Verification items for the finished model (mm, model axes). Face numbers are marked on the shaded views. A direction names the side the tool comes from. Give positions to 0.01 mm unless a question says otherwise; leave off trailing zeros. Order: outer loops, then holes, each group sorted by start corner. A loop starts at its lowest first (then second) coordinate and runs counter-clockwise, first axis right, second up. Notation, with made-up numbers: (-25, 24.5) - (24, 24.5) arc R13 ccw to (24, 39.5) - close; hole circle Ø5 at (73.5, -28). An arc over 180 degrees is marked (long way). Answer as a JSON object with one key per item and string values. Group by question number.
(1) Section check A-A (y = 3.5). Record the boundary of the cut face in (x, z), then the cut area to 3 significant figures.
(2) Mould release check, pull along Y, two halves, no side actions. Record for the marked faces 4, 5, 6 and 7: +Y half, -Y half, draft (parallel to the pull), parting line (faces both ways), or undercut.
(3) Depth check by flat-ended pin: pin 1 Ø12 at (y, z) = (18, -13.5) entering from +X; pin 2 Ø1.5 at (x, y) = (5, -15) entering from +Z; pin 3 Ø0.9 at (y, z) = (13, -18) entering from -X; pin 4 Ø3.5 at (x, y) = (-17.5, 13.5) entering from -Z. Enter the tip coordinate at first touch or a pass-through.
(4) Thickness scan on line 1 (X direction, y = -29, z = -12); line 2 (Z direction, x = 15, y = -28); line 3 (X direction, y = -29, z = -14). Record the ranges inside material, lowest first.
(5) Section check B-B (y = -48). Record the boundary of the cut face in (x, z), then the cut area to 3 significant figures.
(6) Access from +Z, -Z, +X, -X, +Y, -Y to the whole of each face (thin tool, end or side, straight path). Record for the marked faces 1, 2 and 3.
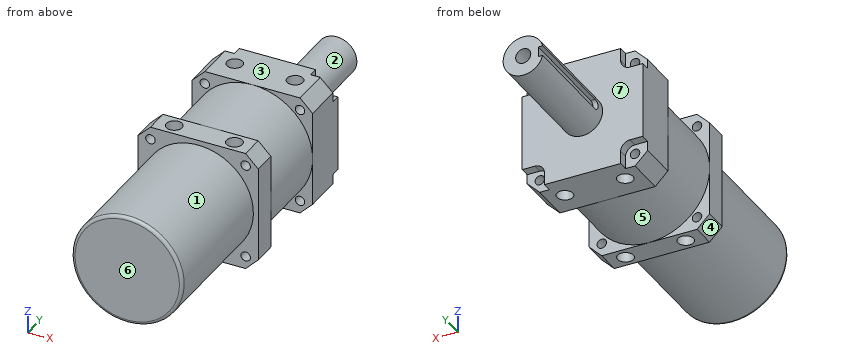
```python
from build123d import *

# Parameters (mm, degrees)
SALIENTE_EXTRUIR1_DEPTH = 15.24
CROQUIS2_R              = 6.35
SALIENTE_EXTRUIR2_DEPTH = 36
CORTAR_EXTRUIR1_DEPTH   = 1.585
CROQUIS4_R              = 1.5
CORTAR_EXTRUIR2_DEPTH   = 58.890781738
CROQUIS5_R              = 19.05
SALIENTE_EXTRUIR3_DEPTH = 25.4
SALIENTE_EXTRUIR4_START = 7.62
CROQUIS6_R              = 1.5
SALIENTE_EXTRUIR4_DEPTH = 7.62
CORTAR_EXTRUIR3_DEPTH   = 3
REDONDEO1_R             = 3
CROQUIS8_R              = 17.5
SALIENTE_EXTRUIR5_DEPTH = 43
REDONDEO2_R             = 1
CROQUIS9_R              = 2.5
CORTAR_EXTRUIR4_DEPTH   = 10
CORTAR_EXTRUIR5_START   = 28.1
CROQUIS9_2_R            = 2.5
CORTAR_EXTRUIR5_DEPTH   = 10
CROQUIS10_R             = 2.3840625
CORTAR_EXTRUIR6_DEPTH   = 15


with BuildPart() as part:
    # Croquis1 → Saliente-Extruir1 (new body)
    with BuildSketch(Plane(origin=(0, 0, 0), x_dir=(1, 0, 0), z_dir=(0, 1, 0))):
        Polygon((-15.05, 19.05), (-19.05, 15.05), (-19.05, -15.05), (-15.05, -19.05), (15.05, -19.05), (19.05, -15.05), (19.05, 15.05), (15.05, 19.05), align=None)
    extrude(amount=SALIENTE_EXTRUIR1_DEPTH)

    # Croquis2 → Saliente-Extruir2 (add)
    with BuildSketch(Plane(origin=(0, 15.24, 0), x_dir=(1, 0, 0), z_dir=(0, 1, 0))):
        with Locations(Location((0, 0, 0), (0, 0, 270))):
            Circle(CROQUIS2_R)
    extrude(amount=SALIENTE_EXTRUIR2_DEPTH)

    # Croquis3 → Cortar-Extruir1 (cut)
    with BuildSketch(Plane.ZY.offset(6.35)):
        with BuildLine():
            Line((-1.5875, 51.24), (-1.5875, 19.49))
            ThreePointArc((-1.5875, 19.49), (-0.0025, 17.905), (1.5825, 19.49))
            Line((1.5825, 19.49), (1.5825, 51.24))
            Line((1.5825, 51.24), (-1.5875, 51.24))
        make_face()
    extrude(amount=-CORTAR_EXTRUIR1_DEPTH, mode=Mode.SUBTRACT)

    # Croquis4 → Cortar-Extruir2 (cut, through all)
    with BuildSketch(Plane.XZ):
        with Locations(Location((-15.05, -15.05, 0), (0, 0, 270))):
            Circle(CROQUIS4_R)
        with Locations(Location((-15.05, 15.05, 0), (0, 0, 270))):
            Circle(CROQUIS4_R)
        with Locations(Location((15.05, 15.05, 0), (0, 0, 270))):
            Circle(CROQUIS4_R)
        with Locations(Location((15.05, -15.05, 0), (0, 0, 270))):
            Circle(CROQUIS4_R)
    extrude(amount=-CORTAR_EXTRUIR2_DEPTH, mode=Mode.SUBTRACT)

    # Croquis5 → Saliente-Extruir3 (add)
    with BuildSketch(Plane.XZ):
        with Locations(Location((0, 0, 0), (0, 0, 270))):
            Circle(CROQUIS5_R)
    extrude(amount=SALIENTE_EXTRUIR3_DEPTH)

    # Croquis6 → Saliente-Extruir4 (add)
    with BuildSketch(Plane.XZ.offset(25.4).offset(SALIENTE_EXTRUIR4_START)):
        Polygon((-19.05, -15.05), (-15.05, -19.05), (15.05, -19.05), (19.05, -15.05), (19.05, 15.05), (15.05, 19.05), (-15.05, 19.05), (-19.05, 15.05), align=None)
        with Locations(Location((-15.05, 15.05, 0), (0, 0, 270))):
            Circle(CROQUIS6_R, mode=Mode.SUBTRACT)
        with Locations(Location((-15.05, -15.05, 0), (0, 0, 270))):
            Circle(CROQUIS6_R, mode=Mode.SUBTRACT)
        with Locations(Location((15.05, -15.05, 0), (0, 0, 270))):
            Circle(CROQUIS6_R, mode=Mode.SUBTRACT)
        with Locations(Location((15.05, 15.05, 0), (0, 0, 270))):
            Circle(CROQUIS6_R, mode=Mode.SUBTRACT)
    extrude(amount=-SALIENTE_EXTRUIR4_DEPTH)

    # Croquis7 → Cortar-Extruir3 (cut)
    with BuildSketch(Plane(origin=(0, 15.24, 0), x_dir=(1, 0, 0), z_dir=(0, 1, 0))):
        Polygon((-19.05, -12.05), (-12.05, -12.05), (-12.05, -19.05), (-15.05, -19.05), (-19.05, -15.05), align=None)
        Polygon((-12.05, 19.05), (-12.05, 12.05), (-19.05, 12.05), (-19.05, 15.05), (-15.05, 19.05), align=None)
        Polygon((19.05, 12.05), (12.05, 12.05), (12.05, 19.05), (15.05, 19.05), (19.05, 15.05), align=None)
        Polygon((12.05, -19.05), (12.05, -12.05), (19.05, -12.05), (19.05, -15.05), (15.05, -19.05), align=None)
    extrude(amount=-CORTAR_EXTRUIR3_DEPTH, mode=Mode.SUBTRACT)

    # Redondeo1
    redondeo1_edges = [part.edges().sort_by_distance(p)[0] for p in [
        (12.05, 13.74, 12.05),
        (12.05, 13.74, -12.05),
        (-12.05, 13.74, -12.05),
        (-12.05, 13.74, 12.05),
    ]]
    fillet(redondeo1_edges, radius=REDONDEO1_R)

    # Croquis8 → Saliente-Extruir5 (add)
    with BuildSketch(Plane.XZ.offset(33.02)):
        with Locations(Location((0, 0, 0), (0, 0, 270))):
            Circle(CROQUIS8_R)
    extrude(amount=SALIENTE_EXTRUIR5_DEPTH)

    # Redondeo2
    redondeo2_edges = [part.edges().sort_by_distance(p)[0] for p in [
        (0, -76.02, 17.5),
    ]]
    fillet(redondeo2_edges, radius=REDONDEO2_R)

    # Croquis9 → Cortar-Extruir4 (cut)
    with BuildSketch(Plane(origin=(0, 0, 19.05), x_dir=(-1, 0, 0), z_dir=(0, 0, -1))):
        with Locations((9.525, 7.62)):
            Circle(CROQUIS9_R)
        with Locations((-9.525, 7.62)):
            Circle(CROQUIS9_R)
        with Locations((-9.525, -29.21)):
            Circle(CROQUIS9_R)
        with Locations((9.525, -29.21)):
            Circle(CROQUIS9_R)
    extrude(amount=CORTAR_EXTRUIR4_DEPTH, mode=Mode.SUBTRACT)

    # Croquis9<2> → Cortar-Extruir5 (cut)
    with BuildSketch(Plane(origin=(0, 0, 19.05), x_dir=(-1, 0, 0), z_dir=(0, 0, -1)).offset(CORTAR_EXTRUIR5_START)):
        with Locations((9.525, 7.62)):
            Circle(CROQUIS9_2_R)
        with Locations((-9.525, 7.62)):
            Circle(CROQUIS9_2_R)
        with Locations((-9.525, -29.21)):
            Circle(CROQUIS9_2_R)
        with Locations((9.525, -29.21)):
            Circle(CROQUIS9_2_R)
    extrude(amount=CORTAR_EXTRUIR5_DEPTH, mode=Mode.SUBTRACT)

    # Croquis10 → Cortar-Extruir6 (cut)
    with BuildSketch(Plane(origin=(0, 51.24, 0), x_dir=(1, 0, 0), z_dir=(0, 1, 0))):
        with Locations(Location((0, 0, 0), (0, 0, 270))):
            Circle(CROQUIS10_R)
    extrude(amount=-CORTAR_EXTRUIR6_DEPTH, mode=Mode.SUBTRACT)


solid = part.part
```
Solutions:
{
 "1": {"outline": "(-19.05, -15.05) - (-15.05, -19.05) - (15.05, -19.05) - (19.05, -15.05) - (19.05, 15.05) - (15.05, 19.05) - (-15.05, 19.05) - (-19.05, 15.05) - close; hole circle Ø3 at (-15.05, -15.05); hole circle Ø3 at (-15.05, 15.05); hole circle Ø3 at (15.05, -15.05); hole circle Ø3 at (15.05, 15.05)", "area": "1,390 mm2"},
 "2": {"face 4": "draft", "face 5": "undercut", "face 6": "-Y half", "face 7": "+Y half"},
 "3": {"pin 1": "stops at x = 19.05", "pin 2": "stops at z = 18.57", "pin 3": "stops at x = -12.05", "pin 4": "stops at z = -17.81"},
 "4": {"line 1": "x = -19.05 to -12.02, -7.03 to 7.03, 12.02 to 19.05", "line 2": "z = -19.05 to -16.55, -13.55 to 13.55, 16.55 to 19.05", "line 3": "x = -19.05 to -16.12, -13.98 to -12.02, -7.03 to 7.03, 12.02 to 13.98, 16.12 to 19.05"},
 "5": {"outline": "circle Ø35 at (0, 0)", "area": "962 mm2"},
 "6": {"face 1": "-Y", "face 2": "+Y", "face 3": "+Z, +X, -X, +Y, -Y"}
}
